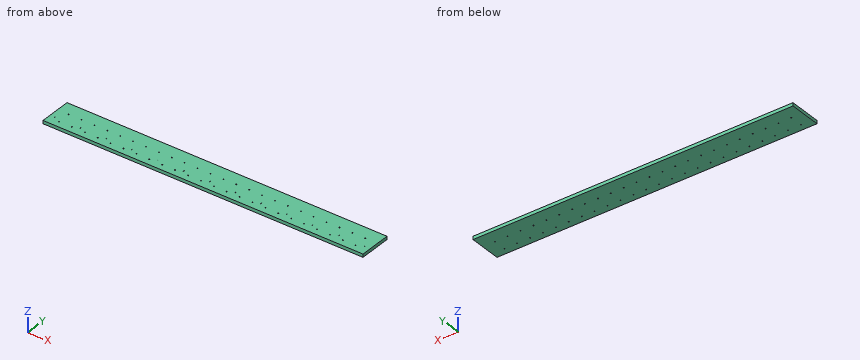
from build123d import *

# Parameters (mm, degrees)
F0_W     = 1000
F0_H     = 100
F1_DEPTH = 10
F2_W     = 0.3
F2_H     = 5
F3_DEPTH = 0.8
F4_R     = 1.5
F5_DEPTH = 10.001


with BuildPart() as f1:
    # F0 (on Top) → F1 (new body)
    with BuildSketch(Plane.XY):
        with Locations((500, 50)):
            Rectangle(F0_W, F0_H)
    extrude(amount=F1_DEPTH)

    # F2 (on face) → F3 (join)
    with BuildSketch(Plane.XY.offset(10)):
        with Locations((15.15, 29.5)):
            Rectangle(F2_W, F2_H)
        with Locations((95.75, 29.5)):
            Rectangle(F2_W, F2_H)
        with Locations((176.35, 29.5)):
            Rectangle(F2_W, F2_H)
        with Locations((256.95, 29.5)):
            Rectangle(F2_W, F2_H)
        with Locations((337.55, 29.5)):
            Rectangle(F2_W, F2_H)
        with Locations((418.15, 29.5)):
            Rectangle(F2_W, F2_H)
        with Locations((498.75, 29.5)):
            Rectangle(F2_W, F2_H)
        with Locations((579.35, 29.5)):
            Rectangle(F2_W, F2_H)
        with Locations((659.95, 29.5)):
            Rectangle(F2_W, F2_H)
        with Locations((740.55, 29.5)):
            Rectangle(F2_W, F2_H)
        with Locations((821.15, 29.5)):
            Rectangle(F2_W, F2_H)
        with Locations((901.75, 29.5)):
            Rectangle(F2_W, F2_H)
        with Locations((982.35, 29.5)):
            Rectangle(F2_W, F2_H)
    extrude(amount=F3_DEPTH)

    # F4 (on face) → F5 (cut, through all)
    with BuildSketch(Plane.XY.offset(10)):
        with Locations((35.3, 20)):
            Circle(F4_R)
        with Locations((75.3, 20)):
            Circle(F4_R)
        with Locations((35.3, 60)):
            Circle(F4_R)
        with Locations((75.3, 60)):
            Circle(F4_R)
        with Locations((115.9, 20)):
            Circle(F4_R)
        with Locations((115.9, 60)):
            Circle(F4_R)
        with Locations((155.9, 60)):
            Circle(F4_R)
        with Locations((155.9, 20)):
            Circle(F4_R)
        with Locations((196.5, 20)):
            Circle(F4_R)
        with Locations((196.5, 60)):
            Circle(F4_R)
        with Locations((236.5, 60)):
            Circle(F4_R)
        with Locations((236.5, 20)):
            Circle(F4_R)
        with Locations((277.1, 20)):
            Circle(F4_R)
        with Locations((277.1, 60)):
            Circle(F4_R)
        with Locations((317.1, 60)):
            Circle(F4_R)
        with Locations((317.1, 20)):
            Circle(F4_R)
        with Locations((357.7, 20)):
            Circle(F4_R)
        with Locations((357.7, 60)):
            Circle(F4_R)
        with Locations((397.7, 60)):
            Circle(F4_R)
        with Locations((397.7, 20)):
            Circle(F4_R)
        with Locations((438.3, 20)):
            Circle(F4_R)
        with Locations((438.3, 60)):
            Circle(F4_R)
        with Locations((478.3, 60)):
            Circle(F4_R)
        with Locations((478.3, 20)):
            Circle(F4_R)
        with Locations((518.9, 20)):
            Circle(F4_R)
        with Locations((518.9, 60)):
            Circle(F4_R)
        with Locations((558.9, 60)):
            Circle(F4_R)
        with Locations((558.9, 20)):
            Circle(F4_R)
        with Locations((599.5, 20)):
            Circle(F4_R)
        with Locations((599.5, 60)):
            Circle(F4_R)
        with Locations((639.5, 60)):
            Circle(F4_R)
        with Locations((639.5, 20)):
            Circle(F4_R)
        with Locations((680.1, 20)):
            Circle(F4_R)
        with Locations((680.1, 60)):
            Circle(F4_R)
        with Locations((720.1, 60)):
            Circle(F4_R)
        with Locations((720.1, 20)):
            Circle(F4_R)
        with Locations((760.7, 20)):
            Circle(F4_R)
        with Locations((760.7, 60)):
            Circle(F4_R)
        with Locations((800.7, 60)):
            Circle(F4_R)
        with Locations((800.7, 20)):
            Circle(F4_R)
        with Locations((841.3, 20)):
            Circle(F4_R)
        with Locations((841.3, 60)):
            Circle(F4_R)
        with Locations((881.3, 60)):
            Circle(F4_R)
        with Locations((881.3, 20)):
            Circle(F4_R)
        with Locations((921.9, 20)):
            Circle(F4_R)
        with Locations((921.9, 60)):
            Circle(F4_R)
        with Locations((961.9, 60)):
            Circle(F4_R)
        with Locations((961.9, 20)):
            Circle(F4_R)
    extrude(amount=-F5_DEPTH, mode=Mode.SUBTRACT)


solid = f1.part
Here's how the part is built. I have some questions about the finished solid (model axes, mm). Round coordinates to 2 decimals unless told otherwise and drop trailing zeros. Order: outer loops, then holes, each group sorted by start corner. A loop starts at its lowest first (then second) coordinate and runs counter-clockwise, first axis right, second up. Notation, with made-up numbers: M -25,68.25 L 27,68.25 A26 cw 27,87.25 Z; hole C -16.5,25 d1. An arc over 180 degrees is marked long. Return JSON: item names as keys, results as strings. Group by question number.
1. I'm going to push flat-ended pins straight in: pin 1 Ø0.9 at (y, z) = (29, 10.5) entering from -X; pin 2 Ø1 at (x, y) = (384.5, 58) entering from +Z; pin 3 Ø12 at (x, y) = (659, 77.5) entering from -Z. Where does each tip first touch, or does it pass through?
2. If we section it at A-A on x = 384: List the corners of the cut face in (y, z) for me, then the cut area to 3 significant figures.
3. Please list where these lines run through material, in increasing order: probe 1 along Y at (x, z) = (961.9, 6.5); probe 2 along Z at (x, y) = (558, 84).
Reply:
{
 "1": {"pin 1": "x = 15", "pin 2": "z = 10", "pin 3": "z = 0"},
 "2": {"outline": "M 0,0 L 100,0 L 100,10 L 0,10 Z", "area": "1,000 mm^2"},
 "3": {"probe 1": "0 to 18.5, 21.5 to 58.5, 61.5 to 100", "probe 2": "0 to 10"}
}
